Source: CAD feature listing. Evaluate the final solid. Frame: model axes, mm. Give positions to 0.01 mm unless a question says otherwise; leave off trailing zeros. Put each result on its own line as item: value.
```python
from build123d import *

# Parameters (mm, degrees)
F0_W          = 12.7
F0_H          = 12.7
F1_DEPTH      = 6.35
F1_DEPTH_BACK = 6.35
F8_D          = 3.683
F8_DEPTH      = 0.254
F8_TIP        = 1.1064848299
F9_D          = 3.683
F9_DEPTH      = 0.254
F9_TIP        = 1.1064848299
F10_D         = 3.683
F10_DEPTH     = 0.254
F10_TIP       = 1.1064848299
F11_D         = 3.683
F11_DEPTH     = 0.254
F11_TIP       = 1.1064848299
F12_D         = 3.683
F12_DEPTH     = 0.254
F12_TIP       = 1.1064848299
F13_D         = 3.683
F13_DEPTH     = 0.254
F13_TIP       = 1.1064848299


with BuildPart() as f1:
    # F0 (on Top) → F1 (new body, two sides)
    with BuildSketch(Plane.XY) as f1_sk:
        Rectangle(F0_W, F0_H)
    extrude(amount=F1_DEPTH)
    extrude(f1_sk.sketch, amount=-F1_DEPTH_BACK)

    # F8
    with Locations(Plane(origin=(0, 6.35, 0), x_dir=(-1, 0, 0), z_dir=(0, 1, 0))):
        with Locations((-4.191, 4.191), (-4.191, 0), (-4.191, -4.191), (4.191, 4.191), (4.191, 0), (4.191, -4.191)):
            Hole(F8_D / 2, depth=F8_DEPTH)
            with Locations((0, 0, -(F8_DEPTH + F8_TIP / 2))):  # 118° drill point
                Cone(0, F8_D / 2, F8_TIP, mode=Mode.SUBTRACT)

    # F9
    with Locations(Plane.YZ.offset(6.35)):
        with Locations((-4.191, 4.191), (-4.191, -4.191), (4.191, 4.191), (4.191, -4.191), (0, 0)):
            Hole(F9_D / 2, depth=F9_DEPTH)
            with Locations((0, 0, -(F9_DEPTH + F9_TIP / 2))):  # 118° drill point
                Cone(0, F9_D / 2, F9_TIP, mode=Mode.SUBTRACT)

    # F10
    with Locations(Plane(origin=(-6.35, 0, 0), x_dir=(0, -1, 0), z_dir=(-1, 0, 0))):
        with Locations((4.191, 4.191), (-4.191, -4.191)):
            Hole(F10_D / 2, depth=F10_DEPTH)
            with Locations((0, 0, -(F10_DEPTH + F10_TIP / 2))):  # 118° drill point
                Cone(0, F10_D / 2, F10_TIP, mode=Mode.SUBTRACT)

    # F11
    with Locations(Plane.XY.offset(6.35)):
        with Locations((4.191, 4.191), (4.191, -4.191), (-4.191, -4.191), (-4.191, 4.191)):
            Hole(F11_D / 2, depth=F11_DEPTH)
            with Locations((0, 0, -(F11_DEPTH + F11_TIP / 2))):  # 118° drill point
                Cone(0, F11_D / 2, F11_TIP, mode=Mode.SUBTRACT)

    # F12
    with Locations(Plane(origin=(0, 0, -6.35), x_dir=(1, 0, 0), z_dir=(0, 0, -1))):
        with Locations((-4.191, 4.191), (0, 0), (4.191, -4.191)):
            Hole(F12_D / 2, depth=F12_DEPTH)
            with Locations((0, 0, -(F12_DEPTH + F12_TIP / 2))):  # 118° drill point
                Cone(0, F12_D / 2, F12_TIP, mode=Mode.SUBTRACT)

    # F13
    with Locations(Plane.XZ.offset(6.35)):
        with Locations((0, 0)):
            Hole(F13_D / 2, depth=F13_DEPTH)
            with Locations((0, 0, -(F13_DEPTH + F13_TIP / 2))):  # 118° drill point
                Cone(0, F13_D / 2, F13_TIP, mode=Mode.SUBTRACT)


solid = f1.part
```
(1) First-contact query: P1, Ø3, axis at x = 4.191, y = -4.191, coming from the +Z side; P2, Ø1.5, axis at x = 3.5, z = 4.5, coming from the +Y side (3 decimals); P3, Ø3.5, axis at y = 4.191, z = -4.191, coming from the -X side. Flat tips, straight axial feed; report the tip coordinate or a pass-through.
Calculated:
P1: stops at z = 5.89
P2: stops at y = 5.895
P3: stops at x = -6.04
(2) Line query: probe 1 along X at (y, z) = (5.5, -0.5); probe 2 along Y at (x, z) = (6.3, 0). Output: solid intervals per line, ascending. Write a range as from..to.
Calculated:
probe 1: x = -6.35..-4.88, -3.5..3.5, 4.88..6.35
probe 2: y = -6.35..-1.84, 1.84..6.35
(3) Section A-A on x = 5.75. Give the number of separate pieces and of enclosed holes in the cut face, then the cut area to 3 significant figures.
Calculated:
separate pieces: 1
enclosed holes: 5
area: 132 mm²
(4) Draft query along Y for faces 1 (the conical face through (5.2, -4, 3.9)), 2 (the flat face through (0, 0, 6.35)), 3 (the conical face through (-4.34, 5.18, 3.91)). Return one class per face: released by +Y, released by -Y, zero draft, split by the parting line, or undercut.
Calculated:
face 1: undercut
face 2: zero draft
face 3: released by +Y
